```python
from build123d import *

# Parameters (mm, degrees)
F1_DEPTH  = 64
F3_DEPTH  = 19
F4_R      = 10
F5_DEPTH  = 19
F6_R      = 19.5
F7_DEPTH  = 12
F8_W      = 83.9615242271
F8_H      = 22
F9_DEPTH  = 6
F10_W     = 22
F10_H     = 56
F11_DEPTH = 6
F12_W     = 70
F12_H     = 25
F13_DEPTH = 25
F15_DEPTH = 70
F16_R     = 7.5
F17_DEPTH = 70
F18_W     = 40
F18_H     = 40.1206766963
F19_DEPTH = 44.501


with BuildPart() as f1:
    # F0 (on Front) → F1 (new body)
    with BuildSketch(Plane.XZ):
        with BuildLine():
            Line((-45, 77.9422863406), (0, 0))
            Line((0, 0), (140, 0))
            Line((140, 0), (140, 19))
            Line((140, 19), (16.7431578065, 19))
            ThreePointArc((16.7431578065, 19), (11.7431578065, 20.3397459622), (8.0829037687, 24))
            Line((8.0829037687, 24), (-14.0455173281, 62.3275496309))
            ThreePointArc((-14.0455173281, 62.3275496309), (-15.0445215531, 69.9157400819), (-10.3852632903, 75.9878036687))
            Line((-10.3852632903, 75.9878036687), (9.5, 87.4685657822))
            Line((9.5, 87.4685657822), (0, 103.9230484541))
            Line((0, 103.9230484541), (-45, 77.9422863406))
        make_face()
    extrude(amount=-F1_DEPTH)

    # F2 (on face) → F3 (join)
    with BuildSketch(Plane(origin=(-45, 0, 77.9422863406), x_dir=(0.8660254038, 0, 0.5), z_dir=(-0.5, 0, 0.8660254038))):
        with BuildLine():
            Line((51.9615242271, 64), (51.9615242271, 0))
            ThreePointArc((51.9615242271, 0), (83.9615242271, 32), (51.9615242271, 64))
        make_face()
    extrude(amount=-F3_DEPTH)

    # F4 (on face) → F5 (cut)
    with BuildSketch(Plane(origin=(-45, 0, 77.9422863406), x_dir=(0.8660254038, 0, 0.5), z_dir=(-0.5, 0, 0.8660254038))):
        with Locations((51.9615242271, 32)):
            Circle(F4_R)
    extrude(amount=-F5_DEPTH, mode=Mode.SUBTRACT)

    # F6 (on face) → F7 (cut)
    with BuildSketch(Plane(origin=(-45, 0, 77.9422863406), x_dir=(0.8660254038, 0, 0.5), z_dir=(-0.5, 0, 0.8660254038))):
        with Locations((51.9615242271, 32)):
            Circle(F6_R)
    extrude(amount=-F7_DEPTH, mode=Mode.SUBTRACT)

    # F8 (on face) → F9 (cut)
    with BuildSketch(Plane(origin=(-45, 0, 77.9422863406), x_dir=(0.8660254038, 0, 0.5), z_dir=(-0.5, 0, 0.8660254038))):
        with Locations((41.9807621135, 32)):
            Rectangle(F8_W, F8_H)
    extrude(amount=-F9_DEPTH, mode=Mode.SUBTRACT)

    # F10 (on face) → F11 (cut)
    with BuildSketch(Plane(origin=(0, 0, 0), x_dir=(0, -1, 0), z_dir=(-0.8660254038, 0, -0.5))):
        with Locations((-32, 62)):
            Rectangle(F10_W, F10_H)
    extrude(amount=-F11_DEPTH, mode=Mode.SUBTRACT)

    # F12 (on face) → F13 (join)
    with BuildSketch(Plane.XY.offset(19)):
        with Locations((90, 32)):
            Rectangle(F12_W, F12_H)
    extrude(amount=F13_DEPTH)

    # F14 (on face) → F15 (join)
    with BuildSketch(Plane.YZ.offset(125)):
        with BuildLine():
            Line((19.5, 44), (44.5, 44))
            ThreePointArc((44.5, 44), (32, 56.5), (19.5, 44))
        make_face()
    extrude(amount=-F15_DEPTH)

    # F16 (on face) → F17 (cut)
    with BuildSketch(Plane.YZ.offset(125)):
        with Locations((32, 44)):
            Circle(F16_R)
    extrude(amount=-F17_DEPTH, mode=Mode.SUBTRACT)

    # F18 (on face) → F19 (cut, through all)
    with BuildSketch(Plane.XZ.offset(-19.5)):
        with Locations((90, 46.0603383482)):
            Rectangle(F18_W, F18_H)
    extrude(amount=-F19_DEPTH, mode=Mode.SUBTRACT)


solid = f1.part
```
CAD build for the part. Positions are in the model's coordinates, mm. A direction names the side the tool comes from. Give positions to 0.01 mm unless a question says otherwise; leave off trailing zeros. Loops run counter-clockwise (first coordinate to the right, second up) from the corner with the lowest first, then second, coordinate; pieces in that order, holes last. Notation, with made-up numbers: (85, -38.75) - (119, -38.75) arc R7 ccw to (119, -32.75) - close; hole circle Ø4 at (81, 74.25). An arc over 180 degrees is marked (long way). Put each result on its own line as item: value.
Q1. Slice it at B-B (y = 10). Give the cut face in (x, z), plus the area to 3 significant figures.
Filled in:
outline: (-45, 77.94) - (0, 0) - (140, 0) - (140, 19) - (16.74, 19) arc R10 cw to (8.08, 24) - (-14.05, 62.33) arc R10 cw to (-10.39, 75.99) - (29.62, 99.09) - (20.12, 115.54) - close
area: 5,260 mm²
Q2. Flat gauge pins, fed straight in: pin 1 (9.5 mm diameter, centred on x = 21.5, z = 110.5, fed in from +Y); pin 2 (2 mm diameter, centred on x = 99, y = 25.5, fed in from +Z); pin 3 (6 mm diameter, centred on y = 43, z = 63, fed in from +X); pin 4 (12.5 mm diameter, centred on x = 101.5, z = 34, fed in from -Y). Where does each tip first touch, or does it go through?
Filled in:
pin 1: stops at y = 59.01
pin 2: stops at z = 26
pin 3: stops at x = -12.7
pin 4: passes through
Q3. Tool access for faces 4 (the face through (89.5, 44.5, 25.8)), 5 (the face through (-14.438, 32.154, 30.924)), 6 (the face through (11.81, 31.55, 20.3)): list every direction of +Z, -Z, +X, -X, +Y, -Y with a clear straight run to the whole face (end or side of a thin tool).
Filled in:
face 4: +Z, +X, +Y
face 5: -X
face 6: +Y, -Y
Q4. Mould opens along Z. For faces 1 (the face through (70, 32, 34)), 2 (the face through (-15.072, 31.552, 69.809)), 3 (the face through (69, 32, 0)) say: pulls with the +Z half, pulls with the -Z half, needs draft (parallel to the pull), parting line crosses it, or undercut.
Filled in:
face 1: needs draft
face 2: undercut
face 3: pulls with the -Z half
Q5. Probe line 1 along Z through (x, y) = (116, 32); line 2 along Y through (x, z) = (69, 44.5); line 3 along X through (y, z) = (38, 21). List the from-to ranges inside material, lowest first.
Filled in:
line 1: z = 0 to 36.5, 51.5 to 56.5
line 2: y = 19.51 to 24.52, 39.48 to 44.49
line 3: x = -12.12 to 10.74, 55 to 125
Q6. Slice it at C-C (y = 32). Give the number of separate pieces and of enclosed holes in the cut face, plus the area to 3 significant figures.
Filled in:
separate pieces: 4
enclosed holes: 0
area: 5,200 mm²
Q7. Slice it at D-D (z = 12.5). Give the cut face in (x, y), plus the area to 3 significant figures.
Filled in:
outline: (-7.22, 0) - (140, 0) - (140, 64) - (-7.22, 64) - close
area: 9,420 mm²
Q8. Slice it at A-A (x = 105). Give the cut face in (y, z).
Filled in:
outline: (0, 0) - (64, 0) - (64, 19) - (44.5, 19) - (44.5, 26) - (19.5, 26) - (19.5, 19) - (0, 19) - close
